Design review of the part built by this model. Coordinates are the model's own, in mm. A direction names the side the tool comes from. Coordinates: 2 decimals unless noted, no trailing zeros. Order: outer loops, then holes, each group sorted by start corner. A loop starts at its lowest first (then second) coordinate and runs counter-clockwise, first axis right, second up. Notation, with made-up numbers: (78, 33.5) -> (89, 33.5) arc R23 cw to (89, 45.5) -> close; hole circle Ø1 at (-28.75, -20). An arc over 180 degrees is marked (long way). Use a Markdown table: item, result. Add a question column.
Q1. Machinability: for faces 1 (the face through (81, -2, 0)), 2 (the face through (39.942, -2, 20)), which of the approach directions +Z, -Z, +X, -X, +Y, -Y give a long, thin tool a straight path to every point of the face, cutting with its end or side? Answer none if there is none.
Q2. Add section B-B (x = 138). State the section outline as (y, z) points.
Q3. Insertion check: pin 1 (8 mm diameter, centred on x = 90, z = 29, fed in from -Y); pin 2 (2.5 mm diameter, centred on y = -1.5, z = 16.5, fed in from +X); pin 3 (1.5 mm diameter, centred on x = 113.5, y = -3, fed in from +Z). Each pin has a flat end and moves straight along its axis. Give the tip position at first contact, or say it passes through.
Q4. The part is to be moulded in two halves that separate along X. For faces 3 (the face through (63, 0, 14)), 4 (the face through (165.1, -2, 5)), 5 (the face through (21.463, -2, 23)), say which applies: pulls with the +X half, pulls with the -X half, needs draft (parallel to the pull), parting line crosses it, or undercut.
Q5. Wall thickness on probe 1 along X at (y, z) = (-3.45, 24); probe 2 along X at (y, z) = (-1.1, 24.5); probe 3 along X at (y, z) = (-1.8, 21): over which ranges is each line inside the solid? List them lowest first.
Q6. Add section A-A (x = 66). State the section outline as (y, z) points.
from build123d import *

# Parameters (mm, degrees)
F1_DEPTH = 4.7625


with BuildPart() as f1:
    # F0 (on Front) → F1 (new body)
    with BuildSketch(Plane.XZ):
        with BuildLine():
            Line((0, 32.512), (0, 0))
            Line((0, 0), (165.1, 0))
            Line((165.1, 0), (165.1, 10.570061))
            ThreePointArc((165.1, 10.570061), (164.670255, 11.729152), (163.588759, 12.327935))
            Line((163.588759, 12.327935), (162.957034, 12.4238))
            ThreePointArc((162.957034, 12.4238), (159.137791, 11.326604), (157.48, 7.715207))
            Line((157.48, 7.715207), (157.48, 6.858))
            ThreePointArc((157.48, 6.858), (156.959236, 5.600764), (155.702, 5.08))
            ThreePointArc((155.702, 5.08), (154.444764, 5.600764), (153.924, 6.858))
            Line((153.924, 6.858), (153.924, 9.700262))
            ThreePointArc((153.924, 9.700262), (152.772897, 12.804971), (149.876034, 14.408855))
            ThreePointArc((149.876034, 14.408855), (146.056791, 13.311659), (144.399, 9.700262))
            Line((144.399, 9.700262), (144.399, 7.493))
            ThreePointArc((144.399, 7.493), (143.841038, 6.145962), (142.494, 5.588))
            ThreePointArc((142.494, 5.588), (141.146962, 6.145962), (140.589, 7.493))
            Line((140.589, 7.493), (140.589, 11.723861))
            ThreePointArc((140.589, 11.723861), (139.437897, 14.82857), (136.541034, 16.432454))
            ThreePointArc((136.541034, 16.432454), (132.721791, 15.335258), (131.064, 11.723861))
            Line((131.064, 11.723861), (131.064, 8.382))
            ThreePointArc((131.064, 8.382), (130.468841, 6.945159), (129.032, 6.35))
            ThreePointArc((129.032, 6.35), (127.595159, 6.945159), (127, 8.382))
            Line((127, 8.382), (127, 13.786005))
            ThreePointArc((127, 13.786005), (125.848897, 16.890714), (122.952034, 18.494598))
            ThreePointArc((122.952034, 18.494598), (119.132791, 17.397402), (117.475, 13.786005))
            Line((117.475, 13.786005), (117.475, 9.017))
            ThreePointArc((117.475, 9.017), (116.842644, 7.490356), (115.316, 6.858))
            ThreePointArc((115.316, 6.858), (113.789356, 7.490356), (113.157, 9.017))
            Line((113.157, 9.017), (113.157, 15.886694))
            ThreePointArc((113.157, 15.886694), (112.005897, 18.991403), (109.109034, 20.595287))
            ThreePointArc((109.109034, 20.595287), (105.289791, 19.49809), (103.632, 15.886694))
            Line((103.632, 15.886694), (103.632, 10.16))
            ThreePointArc((103.632, 10.16), (102.962446, 8.543554), (101.346, 7.874))
            ThreePointArc((101.346, 7.874), (99.729554, 8.543554), (99.06, 10.16))
            Line((99.06, 10.16), (99.06, 18.025927))
            ThreePointArc((99.06, 18.025927), (97.908897, 21.130637), (95.012034, 22.73452))
            ThreePointArc((95.012034, 22.73452), (91.192791, 21.637324), (89.535, 18.025927))
            Line((89.535, 18.025927), (89.535, 10.795))
            ThreePointArc((89.535, 10.795), (88.753854, 8.909146), (86.868, 8.128))
            ThreePointArc((86.868, 8.128), (84.982146, 8.909146), (84.201, 10.795))
            Line((84.201, 10.795), (84.201, 19.59841))
            ThreePointArc((84.201, 19.59841), (82.858046, 23.220571), (79.478372, 25.091768))
            ThreePointArc((79.478372, 25.091768), (75.022589, 23.811706), (73.0885, 19.59841))
            Line((73.0885, 19.59841), (73.0885, 12.319))
            ThreePointArc((73.0885, 12.319), (72.307354, 10.433146), (70.4215, 9.652))
            ThreePointArc((70.4215, 9.652), (68.535646, 10.433146), (67.7545, 12.319))
            Line((67.7545, 12.319), (67.7545, 22.094182))
            ThreePointArc((67.7545, 22.094182), (66.411546, 25.716343), (63.031872, 27.587541))
            ThreePointArc((63.031872, 27.587541), (58.576089, 26.307478), (56.642, 22.094182))
            Line((56.642, 22.094182), (56.642, 12.7))
            ThreePointArc((56.642, 12.7), (55.823656, 10.724344), (53.848, 9.906))
            ThreePointArc((53.848, 9.906), (51.872344, 10.724344), (51.054, 12.7))
            Line((51.054, 12.7), (51.054, 24.628499))
            ThreePointArc((51.054, 24.628499), (49.711046, 28.25066), (46.331372, 30.121858))
            ThreePointArc((46.331372, 30.121858), (41.875589, 28.841796), (39.9415, 24.628499))
            Line((39.9415, 24.628499), (39.9415, 16.129))
            ThreePointArc((39.9415, 16.129), (38.862774, 13.524726), (36.2585, 12.446))
            ThreePointArc((36.2585, 12.446), (33.654226, 13.524726), (32.5755, 16.129))
            Line((32.5755, 16.129), (32.5755, 27.43263))
            ThreePointArc((32.5755, 27.43263), (31.232546, 31.054791), (27.852872, 32.925988))
            ThreePointArc((27.852872, 32.925988), (23.397089, 31.645926), (21.463, 27.43263))
            Line((21.463, 27.43263), (21.463, 17.78))
            ThreePointArc((21.463, 17.78), (20.347077, 15.085923), (17.653, 13.97))
            ThreePointArc((17.653, 13.97), (14.958923, 15.085923), (13.843, 17.78))
            Line((13.843, 17.78), (13.843, 29.49575))
            ThreePointArc((13.843, 29.49575), (12.215612, 33.424612), (8.28675, 35.052))
            Line((8.28675, 35.052), (2.54, 35.052))
            ThreePointArc((2.54, 35.052), (0.743949, 34.308051), (0, 32.512))
        make_face()
    extrude(amount=F1_DEPTH)


solid = f1.part
Established:
| question | item | result |
|---|---|---|
| 1 | face 1 | -Z, +X, -X, +Y, -Y |
| 1 | face 2 | +Z, +Y, -Y |
| 2 | outline | (-4.76, 0) -> (0, 0) -> (0, 15.96) -> (-4.76, 15.96) -> close |
| 3 | pin 1 | through |
| 3 | pin 2 | x = 139.03 |
| 3 | pin 3 | z = 17.81 |
| 4 | face 3 | needs draft |
| 4 | face 4 | pulls with the +X half |
| 4 | face 5 | undercut |
| 5 | probe 1 | 0 to 13.84, 21.46 to 32.58, 39.94 to 51.05, 56.98 to 67.42, 75.25 to 82.04 |
| 5 | probe 2 | 0 to 13.84, 21.46 to 32.58, 39.94 to 51.05, 57.19 to 67.21, 76.03 to 81.26 |
| 5 | probe 3 | 0 to 13.84, 21.46 to 32.58, 39.94 to 51.05, 56.64 to 67.75, 73.27 to 84.02, 90.58 to 98.02 |
| 6 | outline | (-4.76, 0) -> (0, 0) -> (0, 26.15) -> (-4.76, 26.15) -> close |
